Read the model definition and answer for the solid it produces. Units are mm, in the model's axes. A direction names the side the tool comes from. Give positions to 0.01 mm unless a question says otherwise; leave off trailing zeros. Order: outer loops, then holes, each group sorted by start corner. A loop starts at its lowest first (then second) coordinate and runs counter-clockwise, first axis right, second up. Notation, with made-up numbers: M -13.5,-37.75 L -8.5,-37.75 A18 ccw -8.5,-3.75 Z; hole C -14,-36 d5. An arc over 180 degrees is marked long. One line per item, written item: value.
from build123d import *

# Parameters (mm, degrees)
F0_R     = 2
F1_DEPTH = 12
F0_W     = 25
F0_H     = 65
F2_DEPTH = 3
F0_W_2   = 3
F3_DEPTH = 70
F5_DEPTH = 65
F6_R     = 4


with BuildPart() as f1:
    # F0 (on Top) → F1 (new body)
    with BuildSketch(Plane.XY):
        with BuildLine():
            Line((-25.194335, 35.187962), (-28.194335, 35.187962))
            Line((-28.194335, 35.187962), (-28.194335, -29.812038))
            Line((-28.194335, -29.812038), (-25.194335, -29.812038))
            Line((-25.194335, -29.812038), (-25.194335, -25.812038))
            Line((-25.194335, -25.812038), (-23.376417, -25.812038))
            ThreePointArc((-23.376417, -25.812038), (-22.567294, -22.626637), (-19.866929, -24.5))
            ThreePointArc((-19.866929, -24.5), (-19.993566, -25.200365), (-20.35744, -25.812038))
            Line((-20.35744, -25.812038), (-17.194335, -25.812038))
            Line((-17.194335, -25.812038), (-17.194335, -29.812038))
            Line((-17.194335, -29.812038), (-14.194335, -29.812038))
            Line((-14.194335, -29.812038), (-14.194335, 35.187962))
            Line((-14.194335, 35.187962), (-17.194335, 35.187962))
            Line((-17.194335, 35.187962), (-17.194335, 31.187962))
            Line((-17.194335, 31.187962), (-25.194335, 31.187962))
            Line((-25.194335, 31.187962), (-25.194335, 35.187962))
        make_face()
        with Locations((-21.866929, 24.5)):
            Circle(F0_R, mode=Mode.SUBTRACT)
    extrude(amount=F1_DEPTH)

    # F0 (on Top) → F2 (join)
    with BuildSketch(Plane.XY):
        with Locations((-1.694335, 2.687962)):
            Rectangle(F0_W, F0_H)
    extrude(amount=F2_DEPTH)

    # F0 (on Top) → F3 (join)
    with BuildSketch(Plane.XY):
        with Locations((12.305665, 2.687962)):
            Rectangle(F0_W_2, F0_H)
    extrude(amount=F3_DEPTH)

    # F4 (on face) → F5 (join)
    with BuildSketch(Plane.XZ.offset(29.812038)):
        Polygon((10.805665, 70), (13.805665, 70), (13.805665, 73), (-14.194335, 73), (-14.194335, 70), align=None)
    extrude(amount=-F5_DEPTH)

    # F6
    f6_edges = [f1.edges().sort_by_distance(p)[0] for p in [
        (10.805665, 2.687962, 3),
        (10.805665, 2.687962, 70),
        (-14.194335, 2.687962, 3),
        (13.805665, 2.687962, 73),
        (-14.194335, -29.812038, 71.5),
        (-14.194335, 35.187962, 71.5),
    ]]
    fillet(f6_edges, radius=F6_R)


solid = f1.part
1) Each of these flat-tipped pins is pushed along its axis until it touches: pin 1 Ø3.5 at (y, z) = (-10, 71) entering from -X; pin 2 Ø17.5 at (y, z) = (8, 24) entering from -X; pin 3 Ø5 at (x, y) = (-21.87, 24.5) entering from +Z. Where does it stop, or does it pass through?
Reported:
pin 1: stops at x = -14.19
pin 2: stops at x = 10.81
pin 3: stops at z = 12
2) Consider probe 1 along X at (y, z) = (-24.5, 8.75); probe 2 along X at (y, z) = (-24.5, 5); probe 3 along Z at (x, y) = (-3, -12). Determine where each line is inside the solid, lowest interval first.
Reported:
probe 1: x = -28.19 to -23.87, -19.87 to -14.19, 10.81 to 13.81
probe 2: x = -28.19 to -23.87, -19.87 to -13.66, 10.27 to 13.81
probe 3: z = 0 to 3, 70 to 73
3) Find section B-B, the plane x = -1. Write down the section's boundary in (y, z).
Reported:
outline: M -29.81,0 L 35.19,0 L 35.19,3 L -29.81,3 Z; M -29.81,70 L 35.19,70 L 35.19,73 L -29.81,73 Z
4) Find section D-D, the plane y = -11.5. Write down the section's boundary in (x, z).
Reported:
outline: M -28.19,0 L 13.81,0 L 13.81,69 A4 ccw 9.81,73 L -14.19,73 L -14.19,70 L 6.81,70 A4 cw 10.81,66 L 10.81,7 A4 cw 6.81,3 L -10.19,3 A4 cw -14.19,7 L -14.19,12 L -28.19,12 Z
5) Find section C-C, the plane y = 24.5. Write down the section's boundary in (x, z).
Reported:
outline: M -28.19,0 L -23.87,0 L -23.87,12 L -28.19,12 Z; M -19.87,0 L 13.81,0 L 13.81,69 A4 ccw 9.81,73 L -14.19,73 L -14.19,70 L 6.81,70 A4 cw 10.81,66 L 10.81,7 A4 cw 6.81,3 L -10.19,3 A4 cw -14.19,7 L -14.19,12 L -19.87,12 Z
6) Determine the mould class of faces 1 (the face through (-2, 3, 3)), 2 (the face through (11, -29.812, 31)), 3 (the face through (-14.194, 2, 9)), 4 (the face through (-2, 2, 73)) for opening direction Z: +Z half, -Z half, draft (parallel to the pull), parting line (faces both ways), or undercut.
Reported:
face 1: undercut
face 2: draft
face 3: undercut
face 4: +Z half
7) Which of the six approach directions +Z, -Z, +X, -X, +Y, -Y give full straight-line access (tool end or side, diameter ignored) to faces 5 (the face through (-19, -25.812, 6)), 6 (the face through (9.6, 3.14, 4.14)), 7 (the face through (-7, 3, 0)), 8 (the face through (-21, 31.188, 6)), 9 (the face through (-14.194, 2, 72))?
Reported:
face 5: +Z, -Z, -Y
face 6: +Y, -Y
face 7: -Z, +X, -X, +Y, -Y
face 8: +Z, -Z, +Y
face 9: +Z, -X, +Y, -Y
8) Find section A-A, the plane z = 8.5. Write down the section's boundary in (x, y), plus the area to 3 significant figures.
Reported:
outline: M -28.19,-29.81 L -25.19,-29.81 L -25.19,-25.81 L -23.38,-25.81 A2 cw long -19.87,-24.5 A2 cw -20.36,-25.81 L -17.19,-25.81 L -17.19,-29.81 L -14.19,-29.81 L -14.19,35.19 L -17.19,35.19 L -17.19,31.19 L -25.19,31.19 L -25.19,35.19 L -28.19,35.19 Z; M 10.81,-29.81 L 13.81,-29.81 L 13.81,35.19 L 10.81,35.19 Z; hole C -21.87,24.5 d4
area: 1,020 mm^2
